Input: part model. Units: mm. Frame: model coordinates. Face numbers are marked on the shaded views. A direction names the side the tool comes from. Give positions to 0.01 mm unless a question says otherwise; leave off trailing zeros. Write each loop counter-clockwise with the first axis right and the second up, starting at its lowest first coordinate (ties: lowest second). Pieces come first, ordered by that corner, then holes. Notation, with made-up numbers: (-32.75, 13) - (-13.75, 13) arc R36 ccw to (-13.75, 48) - close; hole circle Ø1 at (64, 64). An arc over 180 degrees is marked (long way). Use a Markdown table: item, result. Add a question column.
1. Section query B-B, the plane z = -13. Return loops of the section in (x, y).
2. Pin query (flat end, axial travel): pin 1 (0.9 mm diameter, centred on y = 0, z = 0.5, fed in from +X); pin 2 (1.3 mm diameter, centred on y = 0, z = 0.5, fed in from -X); pin 3 (1.5 mm diameter, centred on x = -2, y = 0.5, fed in from -Z). Return the tip coordinate at first contact, or that it passes through.
3. Material intervals for probe 1 along Z at (x, y) = (0, 1); probe 2 along Z at (x, y) = (-1.75, 1.5); probe 3 along Y at (x, z) = (0, -1.75), sorted ascending.
4. Set-up query: the marked faces 1 and 2. Return all of +Z, -Z, +X, -X, +Y, -Y with unobstructed straight access to the full face (end or side cutting, diameter ignored); none if empty.
```python
from build123d import *

# Parameters (mm, degrees)
SKETCH1_R           = 3.375
BOSS_EXTRUDE1_DEPTH = 1.65
SKETCH2_R           = 1.5
BOSS_EXTRUDE2_DEPTH = 23.35
CHAMFER1_SIZE       = 0.3
CUT_EXTRUDE1_DEPTH  = 2
CHAMFER2_SIZE       = 1.65


with BuildPart() as part:
    # Sketch1 → Boss-Extrude1 (new body)
    with BuildSketch(Plane.XY):
        Circle(SKETCH1_R)
    extrude(amount=BOSS_EXTRUDE1_DEPTH)

    # Sketch2 → Boss-Extrude2 (add)
    with BuildSketch(Plane(origin=(0, 0, 0), x_dir=(-1, 0, 0), z_dir=(0, 0, -1))):
        with Locations(Location((0, 0, 0), (0, 0, 180))):
            Circle(SKETCH2_R)
    extrude(amount=BOSS_EXTRUDE2_DEPTH)

    # Chamfer1
    chamfer1_edges = [part.edges().sort_by_distance(p)[0] for p in [
        (-1.5, 0, -23.35),
    ]]
    chamfer(chamfer1_edges, length=CHAMFER1_SIZE)

    # Sketch3 → Cut-Extrude1 (cut)
    with BuildSketch(Plane.XY.offset(1.65)):
        Polygon((0, 1.154700538), (-1, 0.577350269), (-1, -0.577350269), (0, -1.154700538), (1, -0.577350269), (1, 0.577350269), align=None)
    extrude(amount=-CUT_EXTRUDE1_DEPTH, mode=Mode.SUBTRACT)

    # Chamfer2
    chamfer2_edges = [part.edges().sort_by_distance(p)[0] for p in [
        (-3.375, 0, 0),
    ]]
    chamfer(chamfer2_edges, length=CHAMFER2_SIZE - 0.0001)  # a hair under: the kernel refuses the full size


solid = part.part
```
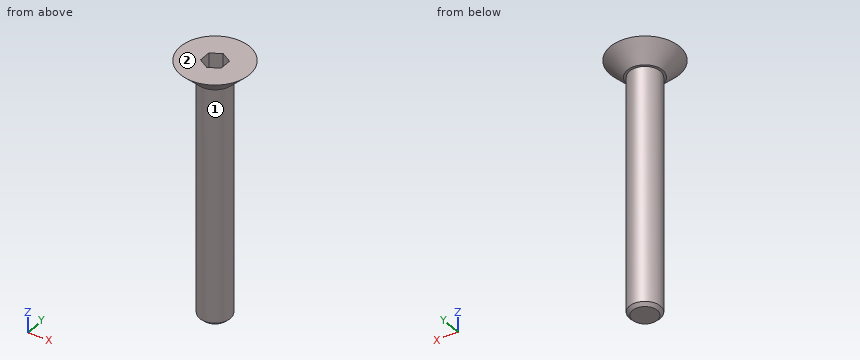
Result sheet:
| question | item | result |
|---|---|---|
| 1 | outline | circle Ø3 at (0, 0) |
| 2 | pin 1 | stops at x = 2.68 |
| 2 | pin 2 | stops at x = -2.88 |
| 2 | pin 3 | stops at z = -23.24 |
| 3 | probe 1 | z = -23.35 to -0.35 |
| 3 | probe 2 | z = 0.58 to 1.65 |
| 3 | probe 3 | y = -1.5 to 1.5 |
| 4 | face 1 | -Z |
| 4 | face 2 | +Z, +X, -X, +Y, -Y |
